Here's how the part is built. I have some questions about the finished solid (model axes, mm). Give positions to 0.01 mm unless a question says otherwise; leave off trailing zeros. Loops run counter-clockwise (first coordinate to the right, second up) from the corner with the lowest first, then second, coordinate; pieces in that order, holes last. Notation, with made-up numbers: (-26.75, 64.5) - (32.25, 64.5) arc R30 cw to (32.25, 102.5) - close; hole circle Ø7 at (-20, -21). An arc over 180 degrees is marked (long way). Use a Markdown table: item, result.
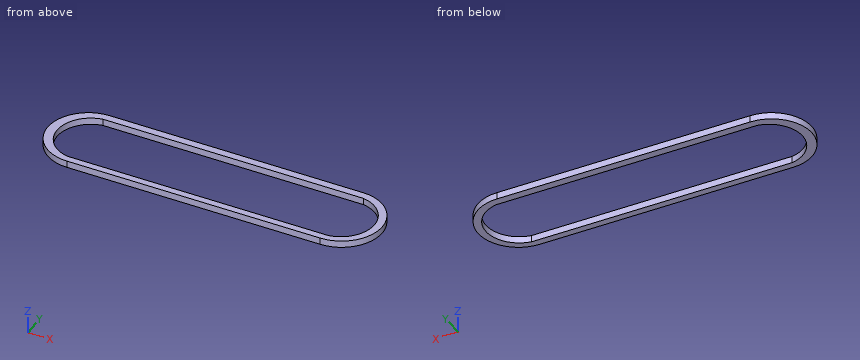
from build123d import *

# Parameters (mm, degrees)
SKETCH_1_W          = 500
SKETCH_1_H          = 120
EXTRUDE_1_DEPTH     = 10
FILLET_8_RADIUS     = 60
FILLET_8_LENGTH     = 10
FILLET_9_RADIUS     = 60
FILLET_9_LENGTH     = 10
CUT_EXTRUDE_1_DEPTH = 10


with BuildPart() as part:
    # 草图1 → 凸台-拉伸1 (new body)
    with BuildSketch(Plane.XY):
        with Locations((176.447257932, 35.78698553)):
            Rectangle(SKETCH_1_W, SKETCH_1_H)
    extrude(amount=EXTRUDE_1_DEPTH)

    # 圆角8: full round fillet: the end face becomes a half cylinder, R = half its width
    fillet_8_face = Plane((-73.552742068, 35.78698553, 5), x_dir=(0, 0, -1), z_dir=(-1, 0, 0))  # on the end face: x along it, z out of the body
    fillet_8_slab = fillet_8_face.offset(-FILLET_8_RADIUS / 2) * Box(FILLET_8_LENGTH, 2 * FILLET_8_RADIUS, FILLET_8_RADIUS, mode=Mode.PRIVATE)  # the body's end, R deep
    fillet_8_round = Plane((-13.552742068, 35.78698553, 5), x_dir=(-1, 0, 0), z_dir=(0, 0, -1)) * Cylinder(FILLET_8_RADIUS, FILLET_8_LENGTH, mode=Mode.PRIVATE)  # its axis R under the face
    add(fillet_8_slab - fillet_8_round, mode=Mode.SUBTRACT)

    # 圆角9: full round fillet: the end face becomes a half cylinder, R = half its width
    fillet_9_face = Plane((426.447257932, 35.78698553, 5), x_dir=(0, 0, 1), z_dir=(1, 0, 0))  # on the end face: x along it, z out of the body
    fillet_9_slab = fillet_9_face.offset(-FILLET_9_RADIUS / 2) * Box(FILLET_9_LENGTH, 2 * FILLET_9_RADIUS, FILLET_9_RADIUS, mode=Mode.PRIVATE)  # the body's end, R deep
    fillet_9_round = Plane((366.447257932, 35.78698553, 5), x_dir=(1, 0, 0), z_dir=(0, 0, 1)) * Cylinder(FILLET_9_RADIUS, FILLET_9_LENGTH, mode=Mode.PRIVATE)  # its axis R under the face
    add(fillet_9_slab - fillet_9_round, mode=Mode.SUBTRACT)

    # 草图4 → 切除-拉伸1 (cut)
    with BuildSketch(Plane.XY.offset(10)):
        with BuildLine():
            Line((-17.715997056, 84.303216301), (373.153004855, 84.303216301))
            ThreePointArc((373.153004855, 84.303216301), (415.190496712, 35.186079817), (373.153004855, -13.931056666))
            Line((373.153004855, -13.931056666), (-17.715997056, -13.931056666))
            ThreePointArc((-17.715997056, -13.931056666), (-59.295663847, 35.186079817), (-17.715997056, 84.303216301))
        make_face()
    extrude(amount=-CUT_EXTRUDE_1_DEPTH, mode=Mode.SUBTRACT)


solid = part.part
(1) Suppose I cut it at A-A on z = 5. Write out the boundary of the cut face in (x, y).
A:
| item | result |
|---|---|
| outline | (-13.55, -24.21) - (366.45, -24.21) arc R60 ccw to (366.45, 95.79) - (-13.55, 95.79) arc R60 ccw to start; hole (-17.72, -13.93) - (373.15, -13.93) arc R49.71 ccw to (373.15, 84.3) - (-17.72, 84.3) arc R49.8 ccw to start |
(2) Suppose I cut it at B-B on x = 333. Write out the boundary of the cut face in (y, z), plus the area to 3 significant figures.
A:
| item | result |
|---|---|
| outline | (-24.21, 0) - (-13.93, 0) - (-13.93, 10) - (-24.21, 10) - close; (84.3, 0) - (95.79, 0) - (95.79, 10) - (84.3, 10) - close |
| area | 218 mm2 |
(3) Will these pins go through, and if not, where does the flat tip stop? pin 1 (1 mm diameter, centred on y = 49, z = 3, fed in from -X); pin 2 (1.5 mm diameter, centred on y = 83.5, z = 4, fed in from -X).
A:
| item | result |
|---|---|
| pin 1 | x = -72.19 |
| pin 2 | x = -50.9 |
(4) If I drill on line 1 (X direction, y = 32.5, z = 7.25); line 2 (Y direction, x = 292, z = 7.25); line 3 (Y direction, x = 370, z = 6.75), over which ranges is the centre line in solid material (lowest first)?
A:
| item | result |
|---|---|
| line 1 | -73.46 to -59.22, 415.12 to 426.36 |
| line 2 | -24.21 to -13.93, 84.3 to 95.79 |
| line 3 | -24.11 to -13.93, 84.3 to 95.68 |
(5) Suppose I cut it at C-C on y = 38.5. Write out the boundary of the cut face in (x, z).
A:
| item | result |
|---|---|
| outline | (-73.49, 0) - (-59.19, 0) - (-59.19, 10) - (-73.49, 10) - close; (415.08, 0) - (426.39, 0) - (426.39, 10) - (415.08, 10) - close |
